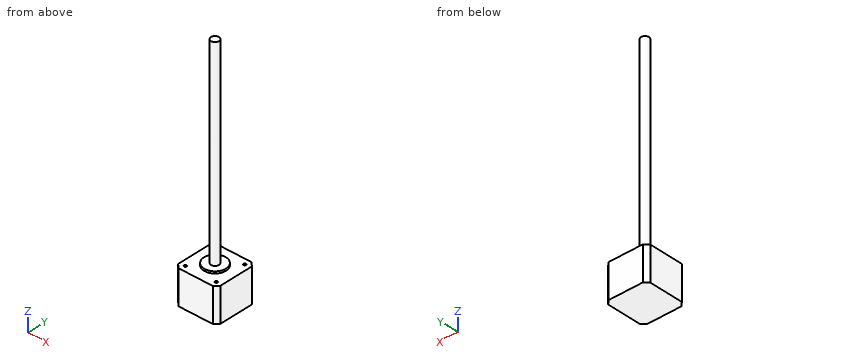
from build123d import *

# Parameters (mm, degrees)
SKETCH1_W           = 42.3
SKETCH1_H           = 42.3
BOSS_EXTRUDE1_DEPTH = 34
SKETCH2_R           = 11
BOSS_EXTRUDE2_DEPTH = 2
SKETCH3_R           = 4
BOSS_EXTRUDE3_DEPTH = 200
CHAMFER1_SIZE       = 4
SKETCH4_R           = 1.25
CUT_EXTRUDE1_DEPTH  = 10


with BuildPart() as part:
    # Sketch1 → Boss-Extrude1 (new body)
    with BuildSketch(Plane.XY):
        Rectangle(SKETCH1_W, SKETCH1_H)
    extrude(amount=BOSS_EXTRUDE1_DEPTH)

    # Sketch2 → Boss-Extrude2 (add)
    with BuildSketch(Plane.XY.offset(34)):
        Circle(SKETCH2_R)
    extrude(amount=BOSS_EXTRUDE2_DEPTH)

    # Sketch3 → Boss-Extrude3 (add)
    with BuildSketch(Plane.XY.offset(36)):
        Circle(SKETCH3_R)
    extrude(amount=BOSS_EXTRUDE3_DEPTH)

    # Chamfer1
    chamfer1_edges = [part.edges().sort_by_distance(p)[0] for p in [
        (21.15, -21.15, 17),
        (-21.15, -21.15, 17),
        (-21.15, 21.15, 17),
        (21.15, 21.15, 17),
    ]]
    chamfer(chamfer1_edges, length=CHAMFER1_SIZE)

    # Sketch4 → Cut-Extrude1 (cut)
    with BuildSketch(Plane.XY.offset(34)):
        with Locations((-15.5, 15.5)):
            Circle(SKETCH4_R)
        with Locations((15.5, 15.5)):
            Circle(SKETCH4_R)
        with Locations((15.5, -15.5)):
            Circle(SKETCH4_R)
        with Locations((-15.5, -15.5)):
            Circle(SKETCH4_R)
    extrude(amount=-CUT_EXTRUDE1_DEPTH, mode=Mode.SUBTRACT)


solid = part.part
Input: part model. Units: mm. Frame: model coordinates. Round coordinates to 2 decimals unless told otherwise and drop trailing zeros. Loops run counter-clockwise (first coordinate to the right, second up) from the corner with the lowest first, then second, coordinate; pieces in that order, holes last. Notation, with made-up numbers: (29.5, 13) -> (67.5, 13) arc R14 cw to (67.5, 20) -> close; hole circle Ø10 at (38, 4.5). An arc over 180 degrees is marked (long way). Answer as a JSON object with one key per item and string values. Group by question number.
1) Pin query (flat end, axial travel): pin 1 (0.8 mm diameter, centred on x = 15, y = -15, fed in from +Z); pin 2 (3 mm diameter, centred on x = 15.5, y = -15.5, fed in from +Z); pin 3 (6 mm diameter, centred on x = 5.5, y = 9, fed in from +Z). Return the tip coordinate at first contact, or that it passes through.
2) Section query B-B on y = -6. Output: boundary loops of the cut face in (x, z), plus the area to 3 significant figures.
3) Ray query, L1, parallel to Y at x = 15.5, z = 29; L2, parallel to Z at x = -4.5, y = 5.5; L3, parallel to Z at x = 13.5, y = 14. Return the intervals inside material, ascending.
4) Section query A-A on x = 0. Output: boundary loops of the cut face in (y, z).
5) Section query C-C on z = 84. Output: boundary loops of the cut face in (x, y).
Reply:
{
 "1": {"pin 1": "stops at z = 24", "pin 2": "stops at z = 34", "pin 3": "stops at z = 36"},
 "2": {"outline": "(-21.15, 0) -> (21.15, 0) -> (21.15, 34) -> (9.22, 34) -> (9.22, 36) -> (-9.22, 36) -> (-9.22, 34) -> (-21.15, 34) -> close", "area": "1,480 mm2"},
 "3": {"L1": "y = -21.15 to -16.75, -14.25 to 14.25, 16.75 to 21.15", "L2": "z = 0 to 36", "L3": "z = 0 to 34"},
 "4": {"outline": "(-21.15, 0) -> (21.15, 0) -> (21.15, 34) -> (11, 34) -> (11, 36) -> (4, 36) -> (4, 236) -> (-4, 236) -> (-4, 36) -> (-11, 36) -> (-11, 34) -> (-21.15, 34) -> close"},
 "5": {"outline": "circle Ø8 at (0, 0)"}
}
